Could you check a few things on this model? Use its own coordinates, in mm. A direction names the side the tool comes from. Give positions to 0.01 mm unless a question says otherwise; leave off trailing zeros. Write each loop counter-clockwise with the first axis right and the second up, starting at its lowest first coordinate (ties: lowest second). Pieces come first, ordered by that corner, then holes. Notation, with made-up numbers: M 71.25,-18 L 117.25,-18 A35 cw 117.25,16 Z; hole C 83,25 d4. An arc over 180 degrees is marked long. Write each question's results on one line, items separated by ' | '. Start each with the question number.
from build123d import *

# Parameters (mm, degrees)
SKETCH1_W            = 115
SKETCH1_H            = 80
BOSS_EXTRUDE1_DEPTH  = 10
SKETCH2_R            = 2.5
CUT_EXTRUDE1_DEPTH   = 10
LPATTERN1_COUNT      = 2
LPATTERN1_PITCH      = 79.8
LPATTERN1_COUNT_DIR2 = 2
LPATTERN1_PITCH_DIR2 = 30
SKETCH4_R            = 5
CUT_EXTRUDE2_DEPTH   = 3
LPATTERN2_COUNT      = 2
LPATTERN2_PITCH      = 79.8
LPATTERN2_COUNT_DIR2 = 2
LPATTERN2_PITCH_DIR2 = 30
SKETCH5_R            = 2.5
CUT_EXTRUDE3_DEPTH   = 11
SKETCH6_R            = 5
CUT_EXTRUDE4_DEPTH   = 3


with BuildPart() as part:
    # Sketch1 → Boss-Extrude1 (new body)
    with BuildSketch(Plane.XY):
        Rectangle(SKETCH1_W, SKETCH1_H)
    extrude(amount=BOSS_EXTRUDE1_DEPTH)

    # Sketch2 → Cut-Extrude1 (cut)
    with BuildSketch(Plane.XY.offset(10)):
        with Locations((-39.9, 27.5)):
            Circle(SKETCH2_R)
    cut_extrude1 = extrude(amount=-CUT_EXTRUDE1_DEPTH, mode=Mode.SUBTRACT)

    # LPattern1: Cut-Extrude1 2 × 2
    with Locations(*[(i * LPATTERN1_PITCH, -j * LPATTERN1_PITCH_DIR2, 0) for i in range(LPATTERN1_COUNT) for j in range(LPATTERN1_COUNT_DIR2) if (i, j) != (0, 0)]):
        add(cut_extrude1, mode=Mode.SUBTRACT)

    # Sketch4 → Cut-Extrude2 (cut)
    with BuildSketch(Plane.XY.offset(10)):
        with Locations((-39.9, 27.5)):
            Circle(SKETCH4_R)
    cut_extrude2 = extrude(amount=-CUT_EXTRUDE2_DEPTH, mode=Mode.SUBTRACT)

    # LPattern2: Cut-Extrude2 2 × 2
    with Locations(*[(i * LPATTERN2_PITCH, -j * LPATTERN2_PITCH_DIR2, 0) for i in range(LPATTERN2_COUNT) for j in range(LPATTERN2_COUNT_DIR2) if (i, j) != (0, 0)]):
        add(cut_extrude2, mode=Mode.SUBTRACT)

    # Sketch5 → Cut-Extrude3 (cut, through all)
    with BuildSketch(Plane.XY.offset(10)):
        with Locations((0, -21.009684694)):
            Circle(SKETCH5_R)
    extrude(amount=-CUT_EXTRUDE3_DEPTH, mode=Mode.SUBTRACT)

    # Sketch6 → Cut-Extrude4 (cut)
    with BuildSketch(Plane.XY.offset(10)):
        with Locations((0, -21.009684694)):
            Circle(SKETCH6_R)
    extrude(amount=-CUT_EXTRUDE4_DEPTH, mode=Mode.SUBTRACT)


solid = part.part
Q1. If we section it at B-B (y = -2.5): Please give me the cut outline in (x, z), plus the area to 3 significant figures.
Q2. I'm going to push a flat-ended pin straight in: P1, Ø3, axis at x = 2.5, y = -21, coming from the +Z side. Where does the tip first touch, or does it pass through?
Q3. For faces 4 (the face through (-39, 30, 7)), 5 (the face through (1.34, -18.9, 3.55)), which set-ups out of +Z, -Z, +X, -X, +Y, -Y let a thin tool reach every point of the face, with its end or its side?
Q4. Please list where these lines run through material, in increasing order: line 1 (Y direction, x = -39.9, z = 9.25); line 2 (X direction, y = 31.5, z = 8.75); line 3 (X direction, y = -2, z = 3.75). Write a range as [from, to].
Q5. If we mould it in two halves opening along Y, with no side actions, what happens to faces 1 (the face through (-1, 40, 5)), 2 (the face through (42.207, -6.936, 8.521)), 3 (the face through (-57.5, -1, 5))? For each: pulls with the +Y half, pulls with the -Y half, needs draft (parallel to the pull), parting line crosses it, or undercut.
Q6. If we section it at C-C (x = 0): Please give me the cut outline in (y, z), plus the area to 3 significant figures.
Q7. If we section it at A-A (x = -39.9): Please give me the cut outline in (y, z), plus the area to 3 significant figures.
Determined:
1) outline: M -57.5,0 L -42.4,0 L -42.4,7 L -44.9,7 L -44.9,10 L -57.5,10 Z; M -37.4,0 L 37.4,0 L 37.4,7 L 34.9,7 L 34.9,10 L -34.9,10 L -34.9,7 L -37.4,7 Z; M 42.4,0 L 57.5,0 L 57.5,10 L 44.9,10 L 44.9,7 L 42.4,7 Z | area: 1,020 mm²
2) P1: stops at z = 7
3) face 4: +Z | face 5: +Z, -Z
4) line 1: y = [-40, -7.5], [2.5, 22.5], [32.5, 40] | line 2: x = [-57.5, -42.9], [-36.9, 36.9], [42.9, 57.5] | line 3: x = [-57.5, -42.35], [-37.45, 37.45], [42.35, 57.5]
5) face 1: pulls with the +Y half | face 2: undercut | face 3: needs draft
6) outline: M -40,0 L -23.51,0 L -23.51,7 L -26.01,7 L -26.01,10 L -40,10 Z; M -18.51,0 L 40,0 L 40,10 L -16.01,10 L -16.01,7 L -18.51,7 Z | area: 735 mm²
7) outline: M -40,0 L -5,0 L -5,7 L -7.5,7 L -7.5,10 L -40,10 Z; M 0,0 L 25,0 L 25,7 L 22.5,7 L 22.5,10 L 2.5,10 L 2.5,7 L 0,7 Z; M 30,0 L 40,0 L 40,10 L 32.5,10 L 32.5,7 L 30,7 Z | area: 670 mm²
